Design review of the part built by this model. Coordinates are the model's own, in mm. A direction names the side the tool comes from. Give positions to 0.01 mm unless a question says otherwise; leave off trailing zeros. Loops run counter-clockwise (first coordinate to the right, second up) from the corner with the lowest first, then second, coordinate; pieces in that order, holes last. Notation, with made-up numbers: (50.5, -22.75) -> (87.5, -22.75) arc R5 ccw to (87.5, -18.75) -> close; hole circle Ø4 at (88, -27.5). An arc over 180 degrees is marked (long way). Use a Markdown table: item, result. Add a question column.
1. Add section A-A (y = 0). State the section outline as (x, z) points.
2. Add section B-B (z = 0). State the section outline as (x, y) points, and give its area (3 significant figures).
3. Add section C-C (y = 16.5). State the section outline as (x, z) points, and give its area (3 significant figures).
4. For pin 1 Ø4 at (y, z) = (-6.19, 4.45) entering from +X (1 decimal); pin 2 Ø0.8 at (x, z) = (1, 44) entering from -Y, all flat-tipped, find the tip position at first contact; note any pin that passes through.
5. To check wall thickness, follow line 1 (Z direction, x = 0.7, y = 31); line 2 (Z direction, x = 1.25, y = 29); line 3 (Y direction, x = 0.3, z = -4.5). State the ranges of each line that lie inside material, in increasing order.
6. For faces 1 (the cylindrical face through (0.78, 29.02, 44.51)), 2 (the flat face through (1, 12.827, 45)), list the 3-axis set-ups (+Z, -Z, +X, -X, +Y, -Y) from which the entire face can be reached by the end or side of a thin tool; tool diameter is ignored.
7. Draft analysis for pull direction Z (two halves, no side actions). For faces 3 (the flat face through (1.588, 17, 25)), 4 (the cylindrical face through (0.783, 17.626, 37.483)), 5 (the cylindrical face through (0.78, -6.75, -10.76)), 6 (the cylindrical face through (0.783, 28.894, 53.638)), state which applies: pulls with the +Z half, pulls with the -Z half, needs draft (parallel to the pull), parting line crosses it, or undercut.
8. Add section D-D (x = 1.3). Count the separate pieces of the cut face and the enclosed holes in it, and give its area (3 significant figures).
Autodesk Inventor part; units mm, degrees
ref_plane "YZ Plane" through (0, 0, 0) normal (1, 0, 0) x (0, 1, 0)
ref_plane "XZ Plane" through (0, 0, 0) normal (0, 1, 0) x (-1, 0, 0)
ref_plane "XY Plane" through (0, 0, 0) normal (0, 0, 1) x (1, 0, 0)
sketch "Sketch1" plane through (0, 0, 0) normal (1, 0, 0) x (0, 1, 0)
  circle A0 centre (0, 0) radius 2.159
  line L0 (0, 0) -> (0, 39.624) construction
  line L1 (0, 39.624) -> (12.827, 39.624) construction
  line L2 (12.827, 39.624) -> (12.827, 51.054)
  circle A1 centre (0, 0) radius 12.7
  line L3 (12.827, 39.624) -> (-10.3145, 7.4095)
  line L4 (12.827, 51.054) -> (35.687, 51.054) construction
  line L5 (35.687, 51.054) -> (35.687, 34.544)
  line L6 (35.687, 34.544) -> (12.827, 34.544) construction
  line L7 (12.827, 34.544) -> (12.827, 51.054)
  line L8 (35.687, 34.544) -> (10.8726, -6.5633)
  circle A2 centre (30.607, 45.974) radius 2.159
  line L9 (30.607, 45.974) -> (30.607, 33.274) construction
  line L10 (30.607, 45.974) -> (17.907, 45.974) construction
  circle A3 centre (30.607, 39.624) radius 2.159
  circle A4 centre (17.907, 45.974) radius 2.159
  circle A5 centre (17.907, 39.624) radius 2.159
  line L11 (12.827, 51.054) -> (35.687, 64.2522)
  line L12 (35.687, 64.2522) -> (35.687, 51.054)
  circle A6 centre (30.607, 52.324) radius 2.159
  circle A7 centre (6.1887, -4.4457) radius 2.159
  line L13 (0, 0) -> (6.1887, -4.4457) construction
  circle A8 centre (0, 0) radius 7.62 construction
  circle A9 centre (-6.1887, 4.4457) radius 2.159
  dimension "d29" = 15.24
  dimension "d0" = 4.318
  dimension "d1" = 39.624
  dimension "d2" = 11.43
  dimension "d3" = 12.827
  dimension "d5" = 25.4
  dimension "d6" = 22.86
  dimension "d7" = 16.51
  dimension "d8" = 4.318
  dimension "d9" = 5.08
  dimension "d10" = 5.08
  dimension "d11" = 12.7
  dimension "d12" = 12.7
  dimension "d15" = 6.35
  dimension "d18" = 12.7
  dimension "d21" = 30
  dimension "d22" = 6.35
  dimension "d26" = 4.318
  dimension "d32" = 360
extrude "Extrusion1" add sketch "Sketch1" along normal blind 1.5875
fillet "Fillet1" radius 3.175 4 edges at (0.7937, 12.827, 39.624) (0.7937, 35.687, 34.544) (0.7937, 35.687, 64.2522) (0.7937, 12.827, 51.054)
properties part number "IntakeArm" material "Aluminum 6061"
Taken from the geometry:
| question | item | result |
|---|---|---|
| 1 | outline | (0, -12.7) -> (1.59, -12.7) -> (1.59, -2.16) -> (0, -2.16) -> close; (0, 2.16) -> (1.59, 2.16) -> (1.59, 21.77) -> (0, 21.77) -> close |
| 2 | outline | (0, -12.7) -> (1.59, -12.7) -> (1.59, -2.16) -> (0, -2.16) -> close; (0, 2.16) -> (1.59, 2.16) -> (1.59, 14.83) -> (0, 14.83) -> close |
| 2 | area | 36.9 mm^2 |
| 3 | outline | (0, 2.76) -> (1.59, 2.76) -> (1.59, 37.99) -> (0, 37.99) -> close; (0, 41.26) -> (1.59, 41.26) -> (1.59, 44.34) -> (0, 44.34) -> close; (0, 47.61) -> (1.59, 47.61) -> (1.59, 53.17) -> (0, 53.17) -> close |
| 3 | area | 69.6 mm^2 |
| 4 | pin 1 | passes through |
| 4 | pin 2 | stops at y = 12.83 |
| 5 | line 1 | z = 26.78 to 37.5, 41.75 to 43.85, 48.1 to 50.2, 54.45 to 61.54 |
| 5 | line 2 | z = 23.47 to 38.18, 41.07 to 44.53, 47.42 to 50.88, 53.77 to 60.39 |
| 5 | line 3 | y = -11.88 to 4.03, 8.35 to 12.12 |
| 6 | face 1 | +X, -X |
| 6 | face 2 | +Z, +X, -X, -Y |
| 7 | face 3 | needs draft |
| 7 | face 4 | undercut |
| 7 | face 5 | parting line crosses it |
| 7 | face 6 | undercut |
| 8 | separate pieces | 1 |
| 8 | enclosed holes | 8 |
| 8 | area | 1,650 mm^2 |
